Source: CAD feature listing. Evaluate the final solid. Frame: model axes, mm. Coordinates: 2 decimals unless noted, no trailing zeros. Order: outer loops, then holes, each group sorted by start corner. A loop starts at its lowest first (then second) coordinate and runs counter-clockwise, first axis right, second up.
```python
from build123d import *

# Parameters (mm, degrees)
F_5_0MM_DOWEL_HOLE1_D               = 5.2
F_5_0MM_DOWEL_HOLE1_DEPTH           = 5
F_5_0MM_DOWEL_HOLE1_TIP             = 1.562237609
F_5_0MM_DOWEL_HOLE1_ON_FACE_2_D     = 5.2
F_5_0MM_DOWEL_HOLE1_ON_FACE_2_DEPTH = 5
F_5_0MM_DOWEL_HOLE1_ON_FACE_2_TIP   = 1.562237609


with BuildPart() as part:
    # Sweep1: sweep along a path in Sketch2
    with BuildLine(Plane(origin=(0, 0, 0), x_dir=(1, 0, 0), z_dir=(0, 1, 0))) as sweep1_path:
        ThreePointArc((44.295, 25.573730174), (14.765, 25.573730174), (0, 0))
    # Sketch1 → Sweep1 (sweep)
    with BuildSketch(Plane.XY):
        with BuildLine():
            Line((0.5, 16.097236564), (0.5, 13.550778575))
            ThreePointArc((0.5, 13.550778575), (13.56, 0), (0.5, -13.550778575))
            Line((0.5, -13.550778575), (0.5, -16.097236564))
            ThreePointArc((0.5, -16.097236564), (16.105, 0), (0.5, 16.097236564))
        make_face()
    sweep(path=sweep1_path.line)

    # Ø5.0mm Dowel Hole1
    with Locations(Plane(origin=(29.53, 0, -13.425), x_dir=(1, 0, 0), z_dir=(0, 0, 1))):
        with Locations((0, 0)):
            Hole(F_5_0MM_DOWEL_HOLE1_D / 2, depth=F_5_0MM_DOWEL_HOLE1_DEPTH)
            with Locations((0, 0, -(F_5_0MM_DOWEL_HOLE1_DEPTH + F_5_0MM_DOWEL_HOLE1_TIP / 2))):  # 118° drill point
                Cone(0, F_5_0MM_DOWEL_HOLE1_D / 2, F_5_0MM_DOWEL_HOLE1_TIP, mode=Mode.SUBTRACT)

    # Ø5.0mm Dowel Hole1 on face 2
    with Locations(Plane(origin=(17.903608954, 0, -6.7125), x_dir=(-0.500000174844, 0, 0.866025302838), z_dir=(0.866025302838, 0, 0.500000174844))):
        with Locations((0, 0)):
            Hole(F_5_0MM_DOWEL_HOLE1_ON_FACE_2_D / 2, depth=F_5_0MM_DOWEL_HOLE1_ON_FACE_2_DEPTH)
            with Locations((0, 0, -(F_5_0MM_DOWEL_HOLE1_ON_FACE_2_DEPTH + F_5_0MM_DOWEL_HOLE1_ON_FACE_2_TIP / 2))):  # 118° drill point
                Cone(0, F_5_0MM_DOWEL_HOLE1_ON_FACE_2_D / 2, F_5_0MM_DOWEL_HOLE1_ON_FACE_2_TIP, mode=Mode.SUBTRACT)


solid = part.part
```
1. Draft query along Y for faces 1 (the face through (37.525, 2.31, -13.847)), 2 (the face through (27.13, -1, -14.72)). Return one class per face: released by +Y, released by -Y, zero draft, split by the parting line, or undercut.
Findings:
face 1: zero draft
face 2: undercut
2. Section query B-B on y = 6.5. Return loops of the section in (x, z), plus the area to 3 significant figures.
Findings:
outline: (11.9, 0) arc R17.63 ccw to (38.34, -15.27) - (36.93, -12.81) arc R14.79 cw to (14.74, 0) - close
area: 96.2 mm2
3. Pin query (flat end, axial travel): P1, Ø12, axis at x = 11, z = -18.5, coming from the -Y side; P2, Ø8, axis at x = 23.5, z = -14.5, coming from the -Y side; P3, Ø5, axis at x = 36.5, y = 2.5, coming from the +Z side; P4, Ø1.5, axis at y = -8, z = -7, coming from the -X side. Return the tip coordinate at first contact, or that it passes through.
Findings:
P1: stops at y = -16.1
P2: stops at y = -12.76
P3: stops at z = -11.63
P4: stops at x = 11.62
4. Section query A-A on y = 0. Count the separate pieces of the cut face and the enclosed holes in it, plus the area to 3 significant figures.
Findings:
separate pieces: 3
enclosed holes: 0
area: 51.7 mm2
5. Section query C-C on y = -7. Return loops of the section in (x, z), plus the area to 3 significant figures.
Findings:
outline: (11.61, 0) arc R17.92 ccw to (38.49, -15.52) - (37.04, -13.01) arc R15.03 cw to (14.5, 0) - close
area: 99.7 mm2
6. Ray query, line 1 (Y direction, x = 14, z = -20.5); line 2 (Y direction, x = 17, z = -12.25); line 3 (X direction, y = 0, z = -14.75). Return the intervals inside material, ascending.
Findings:
line 1: y = -15.65 to -13.01, 13.01 to 15.65
line 2: y = -10.73 to -6.3, 6.3 to 10.73
line 3: x = 23.41 to 26.93, 32.13 to 35.65
